The model under review builds one solid part; all positions refer to its coordinate system, in mm. A direction names the side the tool comes from. Coordinates: 2 decimals unless noted, no trailing zeros. Write each loop counter-clockwise with the first axis right and the second up, starting at its lowest first coordinate (ties: lowest second). Pieces come first, ordered by that corner, then holes. Notation, with made-up numbers: (59, -12) - (98, -12) arc R24 cw to (98, 24) - close; hole circle Ø7 at (41.5, 21). An arc over 180 degrees is marked (long way). Return JSON: item names as keys, results as strings. Group by question number.
(1) We need section B-B on y = 15.5. State the section outline as (x, z) points, then the cut area to 3 significant figures.
(2) To check wall thickness, follow L1, parallel to Y at x = 16.5, z = -15; L2, parallel to X at y = -25.5, z = -16; L3, parallel to X at y = -27.5, z = -4. State the ranges of each line that lie inside material, in increasing order. Write a range as from..to.
(3) We need section C-C on x = -16. State the section outline as (y, z) points.
(4) Draft analysis for pull direction X (two halves, no side actions). For faces 1 (the face through (18, -18, -18.102)), 2 (the face through (2.933, 0, 19)), 3 (the face through (-1.215, 25, 0)), state which applies: released by +X, released by -X, zero draft, split by the parting line, or undercut.
(5) Tool access review of faces 4 (the face through (-16.71, 18.43, -0.25)), 5 (the face through (0, -25, -18.102)), 6 (the face through (0, 2.933, -19)), 7 (the face through (-1.215, -25, 0)), 8 (the face through (25, 0, -18.102)): name each direction out of +Z, -Z, +X, -X, +Y, -Y from which nothing blocks a thin tool from reaching the whole face with its end or side.
(6) For pin 1 Ø4 at (y, z) = (23, -8) entering from +X; pin 2 Ø4 at (x, z) = (20.5, 0.5) entering from -Y; pin 3 Ø0.7 at (x, y) = (-26, 0) entering from -Z; pin 4 Ø1.1 at (y, z) = (0.5, 18.5) entering from -X, all flat-tipped, find the tip position at first contact; note any pin that passes through.
(7) We need section D-D on y = 40. State the section outline as (x, z) points, then the cut area to 3 significant figures.
(8) We need section A-A on z = 1. State the section outline as (x, y) points, then the cut area to 3 significant figures.
```python
from build123d import *

# Parameters (mm, degrees)
F1_DEPTH      = 20.32
F1_DEPTH_BACK = 20.32
F2_W          = 2.4300397955
F2_H          = 36.2040139735
F10_DEPTH     = 44.45
F3_W          = 2.4300397955
F3_H          = 36.2040139735
F11_DEPTH     = 44.45
F4_W          = 2.4300397955
F4_H          = 36.2040139735
F12_DEPTH     = 44.45
F5_W          = 2.4300397955
F5_H          = 36.2040139735
F13_DEPTH     = 44.45
F6_W          = 2.4300397955
F6_H          = 36.2040139735
F14_DEPTH     = 44.45
F9_W          = 2.4300397955
F9_H          = 36.2040139735
F15_DEPTH     = 44.45
F8_W          = 2.4300397955
F8_H          = 36.2040139735
F16_DEPTH     = 44.45
F7_W          = 2.4300397955
F7_H          = 36.2040139735
F17_DEPTH     = 44.45


with BuildPart() as f1:
    # F0 (on Top) → F1 (new body, two sides)
    with BuildSketch(Plane.XY) as f1_sk:
        Polygon((1.2150198978, 2.9333175157), (-1.2150198978, 2.9333175157), (-2.9333175157, 1.2150198978), (-2.9333175157, -1.2150198978), (-1.2150198978, -2.9333175157), (1.2150198978, -2.9333175157), (2.9333175157, -1.2150198978), (2.9333175157, 1.2150198978), align=None)
    extrude(amount=F1_DEPTH)
    extrude(f1_sk.sketch, amount=-F1_DEPTH_BACK)

    # F2 (on face) → F10 (join)
    with BuildSketch(Plane(origin=(0, 2.9333175157, 0), x_dir=(-1, 0, 0), z_dir=(0, 1, 0))):
        Rectangle(F2_W, F2_H)
    extrude(amount=F10_DEPTH)

    # F3 (on face) → F11 (join)
    with BuildSketch(Plane(origin=(2.0741687067, 2.0741687067, 0), x_dir=(-0.7071067812, 0.7071067812, 0), z_dir=(0.7071067812, 0.7071067812, 0))):
        Rectangle(F3_W, F3_H)
    extrude(amount=F11_DEPTH)

    # F4 (on face) → F12 (join)
    with BuildSketch(Plane.YZ.offset(2.9333175157)):
        Rectangle(F4_W, F4_H)
    extrude(amount=F12_DEPTH)

    # F5 (on face) → F13 (join)
    with BuildSketch(Plane(origin=(2.0741687067, -2.0741687067, 0), x_dir=(0.7071067812, 0.7071067812, 0), z_dir=(0.7071067812, -0.7071067812, 0))):
        Rectangle(F5_W, F5_H)
    extrude(amount=F13_DEPTH)

    # F6 (on face) → F14 (join)
    with BuildSketch(Plane.XZ.offset(2.9333175157)):
        Rectangle(F6_W, F6_H)
    extrude(amount=F14_DEPTH)

    # F9 (on face) → F15 (join)
    with BuildSketch(Plane(origin=(-2.0741687067, 2.0741687067, 0), x_dir=(-0.7071067812, -0.7071067812, 0), z_dir=(-0.7071067812, 0.7071067812, 0))):
        Rectangle(F9_W, F9_H)
    extrude(amount=F15_DEPTH)

    # F8 (on face) → F16 (join)
    with BuildSketch(Plane(origin=(-2.9333175157, 0, 0), x_dir=(0, -1, 0), z_dir=(-1, 0, 0))):
        Rectangle(F8_W, F8_H)
    extrude(amount=F16_DEPTH)

    # F7 (on face) → F17 (join)
    with BuildSketch(Plane(origin=(-2.0741687067, -2.0741687067, 0), x_dir=(0.7071067812, -0.7071067812, 0), z_dir=(-0.7071067812, -0.7071067812, 0))):
        Rectangle(F7_W, F7_H)
    extrude(amount=F17_DEPTH)


solid = f1.part
```
Ans:
{
 "1": {"outline": "(-17.22, -18.1) - (-13.78, -18.1) - (-13.78, 18.1) - (-17.22, 18.1) - close; (-1.22, -18.1) - (1.22, -18.1) - (1.22, 18.1) - (-1.22, 18.1) - close; (13.78, -18.1) - (17.22, -18.1) - (17.22, 18.1) - (13.78, 18.1) - close", "area": "337 mm²"},
 "2": {"L1": "-18.22..-14.78, -1.22..1.22, 14.78..18.22", "L2": "-27.22..-23.78, -1.22..1.22, 23.78..27.22", "L3": "-29.22..-25.78, -1.22..1.22, 25.78..29.22"},
 "3": {"outline": "(-17.72, -18.1) - (-14.28, -18.1) - (-14.28, 18.1) - (-17.72, 18.1) - close; (-1.22, -18.1) - (1.22, -18.1) - (1.22, 18.1) - (-1.22, 18.1) - close; (14.28, -18.1) - (17.72, -18.1) - (17.72, 18.1) - (14.28, 18.1) - close"},
 "4": {"face 1": "zero draft", "face 2": "released by +X", "face 3": "undercut"},
 "5": {"face 4": "+Z, -Z, +Y", "face 5": "-Z, +X, -X, -Y", "face 6": "-Z, +X, -X, +Y", "face 7": "+Z, -Z, -Y", "face 8": "-Z, +X, +Y, -Y"},
 "6": {"pin 1": "x = 26.72", "pin 2": "y = -24.22", "pin 3": "z = -18.1", "pin 4": "x = -47.38"},
 "7": {"outline": "(-1.22, -18.1) - (1.22, -18.1) - (1.22, 18.1) - (-1.22, 18.1) - close", "area": "88.0 mm²"},
 "8": {"outline": "(-47.38, -1.22) - (-2.93, -1.22) - (-34.36, -32.65) - (-32.65, -34.36) - (-1.22, -2.93) - (-1.22, -47.38) - (1.22, -47.38) - (1.22, -2.93) - (32.65, -34.36) - (34.36, -32.65) - (2.93, -1.22) - (47.38, -1.22) - (47.38, 1.22) - (2.93, 1.22) - (34.36, 32.65) - (32.65, 34.36) - (1.22, 2.93) - (1.22, 47.38) - (-1.22, 47.38) - (-1.22, 2.93) - (-32.65, 34.36) - (-34.36, 32.65) - (-2.93, 1.22) - (-47.38, 1.22) - close", "area": "893 mm²"}
}
